Build history of the part. All positions in model axes, mm. A direction names the side the tool comes from. Round coordinates to 2 decimals unless told otherwise and drop trailing zeros. Order: outer loops, then holes, each group sorted by start corner. A loop starts at its lowest first (then second) coordinate and runs counter-clockwise, first axis right, second up. Notation, with made-up numbers: (26, 67) -> (33, 67) arc R23 cw to (33, 106) -> close; hole circle Ø11 at (14.5, 88). An arc over 180 degrees is marked (long way). Use a Markdown table: item, result. Add a question column.
Item 1: Slice it at D-D, the plane x = 31. Give the cut face in (y, z).
Item 2: Two-plate mould, pull along X, no slides. Class faces 6 (the face through (-41, 3, 23)), 7 (the face through (-32.35, 10, 37)), 8 (the face through (0, 2, 25.5)), 9 (the face through (41.99, 2.53, 51.25)): released by +X, released by -X, zero draft, split by the parting line, or undercut.
Item 3: Slice it at B-B, the plane z = 46. Give the cut face in (x, y).
Item 4: Slice it at A-A, the plane y = 13.25. Give the cut face in (x, z).
Item 5: 3-axis set-ups, long thin cutter, end or side, ignore diameter. For faces 1 (the face through (41.99, 2.53, 22.25)), 2 (the face through (32.35, 10, 37)), 3 (the face through (-34.35, 10, 37)), 4 (the face through (-42.01, 2.53, 51.25)), 5 (the face through (-25, 2, 38)): which of +Z, -Z, +X, -X, +Y, -Y reach the whole face in a straight line?
Item 6: Pin check, flat tips, straight feed: pin 1 (1.7 mm diameter, centred on x = 39, z = 32.5, fed in from +Y); pin 2 (3 mm diameter, centred on x = -13, z = 25.5, fed in from -Y); pin 3 (5 mm diameter, centred on y = 9.5, z = 35.5, fed in from +X); pin 4 (0.9 mm diameter, centred on y = 2.5, z = 52, fed in from -X). Stop position of each tip, or through.
Item 7: Slice it at C-C, the plane x = -15. Give the cut face in (y, z).
Item 8: Probe L1, parallel to X at y = 1.55, z = 38; L2, parallel to X at y = 12.75, z = 42.5; L3, parallel to Y at x = -41.55, z = 23. List the from-to ranges inside material, lowest first.
from build123d import *

# Parameters (mm, degrees)
SKETCH_1_W          = 86
SKETCH_1_H          = 174
SKETCH_1_W_2        = 50
SKETCH_1_H_2        = 25
SKETCH_1_H_3        = 55
SKETCH_1_W_3        = 76
SKETCH_1_H_4        = 43
EXTRUDE_1_DEPTH     = 5
SKETCH_4_W          = 68.7
SKETCH_4_H          = 115
SKETCH_4_W_2        = 64.7
SKETCH_4_H_2        = 37
SKETCH_4_H_3        = 70
EXTRUDE_2_DEPTH     = 10
SKETCH_5_R          = 0.75
CUT_EXTRUDE_1_DEPTH = 122.783619588
SKETCH_7_W          = 15
SKETCH_7_H          = 8
SKETCH_7_W_2        = 26
SKETCH_7_W_3        = 5
SKETCH_7_H_2        = 10
SKETCH_7_H_3        = 12.119700025
SKETCH_7_W_4        = 6
SKETCH_7_H_4        = 5
SKETCH_7_W_5        = 7
SKETCH_7_H_5        = 21
CUT_EXTRUDE_2_DEPTH = 2
SKETCH_8_R          = 0.75
CUT_EXTRUDE_3_DEPTH = 2
CUT_EXTRUDE_START   = -84
SKETCH_8_3_R        = 0.75
CUT_EXTRUDE_4_DEPTH = 2
SKETCH_9_R          = 0.75
SKETCH_9_W          = 50
SKETCH_9_H          = 55
SKETCH_9_W_2        = 86
SKETCH_9_H_2        = 56
SKETCH_9_W_3        = 76
SKETCH_9_H_3        = 43
CUT_EXTRUDE_5_DEPTH = 123.295748086


with BuildPart() as part:
    # 草图1 → 凸台-拉伸1 (new body)
    with BuildSketch(Plane(origin=(0, 0, 0), x_dir=(1, 0, 0), z_dir=(0, 1, 0))):
        with Locations((0, -26.5)):
            Rectangle(SKETCH_1_W, SKETCH_1_H)
        with Locations((0, -38)):
            Rectangle(SKETCH_1_W_2, SKETCH_1_H_2, mode=Mode.SUBTRACT)
        with Locations((0, 23)):
            Rectangle(SKETCH_1_W_2, SKETCH_1_H_3, mode=Mode.SUBTRACT)
        with Locations((0, -87)):
            Rectangle(SKETCH_1_W_3, SKETCH_1_H_4, mode=Mode.SUBTRACT)
    extrude(amount=EXTRUDE_1_DEPTH)

    # 草图4 → 凸台-拉伸2 (add)
    with BuildSketch(Plane(origin=(0, 5, 0), x_dir=(1, 0, 0), z_dir=(0, 1, 0))):
        Rectangle(SKETCH_4_W, SKETCH_4_H)
        with Locations((0, -37)):
            Rectangle(SKETCH_4_W_2, SKETCH_4_H_2, mode=Mode.SUBTRACT)
        with Locations((0, 20.5)):
            Rectangle(SKETCH_4_W_2, SKETCH_4_H_3, mode=Mode.SUBTRACT)
    extrude(amount=EXTRUDE_2_DEPTH)

    # 草图5 → 切除-拉伸1 (cut, through all)
    with BuildSketch(Plane(origin=(0, 5, 0), x_dir=(1, 0, 0), z_dir=(0, 1, 0))):
        with Locations(Location((-39, 20.5, 0), (0, 0, 270))):
            Circle(SKETCH_5_R)
        with Locations(Location((39, 20.5, 0), (0, 0, 270))):
            Circle(SKETCH_5_R)
        with Locations(Location((-39, -32.5, 0), (0, 0, 270))):
            Circle(SKETCH_5_R)
        with Locations(Location((39, -32.5, 0), (0, 0, 270))):
            Circle(SKETCH_5_R)
        with Locations(Location((-40.1427775, -60.35, 0), (0, 0, 270))):
            Circle(SKETCH_5_R)
        with Locations(Location((40.1427775, -60.35, 0), (0, 0, 270))):
            Circle(SKETCH_5_R)
        with Locations(Location((-40.1427775, -110.530299975, 0), (0, 0, 270))):
            Circle(SKETCH_5_R)
        with Locations(Location((40.1427775, -110.530299975, 0), (0, 0, 270))):
            Circle(SKETCH_5_R)
        with Locations(Location((-40.5, 57.5, 0), (0, 0, 270))):
            Circle(SKETCH_5_R)
        with Locations(Location((-40.5, -38, 0), (0, 0, 270))):
            Circle(SKETCH_5_R)
        with Locations(Location((-40.5, -85.5, 0), (0, 0, 270))):
            Circle(SKETCH_5_R)
        with Locations(Location((40.5, 57.5, 0), (0, 0, 270))):
            Circle(SKETCH_5_R)
        with Locations(Location((40.5, -38, 0), (0, 0, 270))):
            Circle(SKETCH_5_R)
        with Locations(Location((40.5, -85.5, 0), (0, 0, 270))):
            Circle(SKETCH_5_R)
        with Locations(Location((-40.5, -4.5, 0), (0, 0, 270))):
            Circle(SKETCH_5_R)
        with Locations(Location((40.5, -4.5, 0), (0, 0, 270))):
            Circle(SKETCH_5_R)
    extrude(amount=-CUT_EXTRUDE_1_DEPTH, mode=Mode.SUBTRACT)

    # 草图7 → 切除-拉伸2 (cut)
    with BuildSketch(Plane(origin=(0, 5, 0), x_dir=(1, 0, 0), z_dir=(0, 1, 0))):
        with Locations((-24.5, -61.5)):
            Rectangle(SKETCH_7_W, SKETCH_7_H)
        with Locations((0, -61.5)):
            Rectangle(SKETCH_7_W_2, SKETCH_7_H)
        with Locations((-40.5, -78.5)):
            Rectangle(SKETCH_7_W_3, SKETCH_7_H_2)
        with Locations((-40.5, -101.440149988)):
            Rectangle(SKETCH_7_W_3, SKETCH_7_H_3)
        with Locations((-32, -111)):
            Rectangle(SKETCH_7_W_4, SKETCH_7_H_4)
        with Locations((-3, -111)):
            Rectangle(SKETCH_7_W_4, SKETCH_7_H_4)
        with Locations((17.5, -111)):
            Rectangle(SKETCH_7_W_5, SKETCH_7_H_4)
        with Locations((30.5, -111)):
            Rectangle(SKETCH_7_W_5, SKETCH_7_H_4)
        with Locations((40.5, -92)):
            Rectangle(SKETCH_7_W_3, SKETCH_7_H_5)
    extrude(amount=-CUT_EXTRUDE_2_DEPTH, mode=Mode.SUBTRACT)

    # 草图8 → 切除-拉伸3 (cut)
    with BuildSketch(Plane.ZY.offset(43)):
        with Locations((8, 2.5)):
            Circle(SKETCH_8_R)
        with Locations((23, 2.5)):
            Circle(SKETCH_8_R)
        with Locations((52, 2.5)):
            Circle(SKETCH_8_R)
        with Locations((63, 2.5)):
            Circle(SKETCH_8_R)
    extrude(amount=-CUT_EXTRUDE_3_DEPTH, mode=Mode.SUBTRACT)

    # 草图8<3> → 切除-拉伸4 (cut)
    with BuildSketch(Plane.ZY.offset(43).offset(CUT_EXTRUDE_START)):
        with Locations((8, 2.5)):
            Circle(SKETCH_8_3_R)
        with Locations((23, 2.5)):
            Circle(SKETCH_8_3_R)
        with Locations((52, 2.5)):
            Circle(SKETCH_8_3_R)
        with Locations((63, 2.5)):
            Circle(SKETCH_8_3_R)
    extrude(amount=-CUT_EXTRUDE_4_DEPTH, mode=Mode.SUBTRACT)

    # 草图9 → 切除-拉伸5 (cut, through all)
    # profile 1 of 2: a face of its own
    with BuildSketch(Plane(origin=(0, 0, 0), x_dir=(1, 0, 0), z_dir=(0, 1, 0))):
        Polygon((-43, 60.5), (-43, -16.5), (0, -16.5), (43, -16.5), (43, 60.5), align=None)
        with Locations((-40.5, -4.5)):
            Circle(SKETCH_9_R, mode=Mode.SUBTRACT)
        with Locations((-39, 20.5)):
            Circle(SKETCH_9_R, mode=Mode.SUBTRACT)
        with Locations((-40.5, 57.5)):
            Circle(SKETCH_9_R, mode=Mode.SUBTRACT)
        with Locations((0, 23)):
            Rectangle(SKETCH_9_W, SKETCH_9_H, mode=Mode.SUBTRACT)
        with Locations((40.5, -4.5)):
            Circle(SKETCH_9_R, mode=Mode.SUBTRACT)
        with Locations((39, 20.5)):
            Circle(SKETCH_9_R, mode=Mode.SUBTRACT)
        with Locations((40.5, 57.5)):
            Circle(SKETCH_9_R, mode=Mode.SUBTRACT)
    # profile 2 of 2: a face of its own
    with BuildSketch(Plane(origin=(0, 0, 0), x_dir=(1, 0, 0), z_dir=(0, 1, 0))):
        with Locations((0, -85.5)):
            Rectangle(SKETCH_9_W_2, SKETCH_9_H_2)
        with Locations((-40.1427775, -110.530299975)):
            Circle(SKETCH_9_R, mode=Mode.SUBTRACT)
        with Locations((-40.5, -85.5)):
            Circle(SKETCH_9_R, mode=Mode.SUBTRACT)
        with Locations((0, -87)):
            Rectangle(SKETCH_9_W_3, SKETCH_9_H_3, mode=Mode.SUBTRACT)
        with Locations((-40.1427775, -60.35)):
            Circle(SKETCH_9_R, mode=Mode.SUBTRACT)
        with Locations((40.1427775, -110.530299975)):
            Circle(SKETCH_9_R, mode=Mode.SUBTRACT)
        with Locations((40.5, -85.5)):
            Circle(SKETCH_9_R, mode=Mode.SUBTRACT)
        with Locations((40.1427775, -60.35)):
            Circle(SKETCH_9_R, mode=Mode.SUBTRACT)
    extrude(amount=CUT_EXTRUDE_5_DEPTH, mode=Mode.SUBTRACT)


solid = part.part
Check sheet entries:
| question | item | result |
|---|---|---|
| 1 | outline | (0, 16.5) -> (15, 16.5) -> (15, 18.5) -> (5, 18.5) -> (5, 55.5) -> (15, 55.5) -> (15, 57.5) -> (0, 57.5) -> close |
| 2 | face 6 | released by -X |
| 2 | face 7 | undercut |
| 2 | face 8 | undercut |
| 2 | face 9 | zero draft |
| 3 | outline | (-43, 0) -> (-25, 0) -> (-25, 5) -> (-32.35, 5) -> (-32.35, 15) -> (-34.35, 15) -> (-34.35, 5) -> (-43, 5) -> close; (25, 0) -> (43, 0) -> (43, 5) -> (34.35, 5) -> (34.35, 15) -> (32.35, 15) -> (32.35, 5) -> (25, 5) -> close |
| 4 | outline | (-34.35, 16.5) -> (34.35, 16.5) -> (34.35, 57.5) -> (-34.35, 57.5) -> close; hole (-32.35, 18.5) -> (32.35, 18.5) -> (32.35, 55.5) -> (-32.35, 55.5) -> close |
| 5 | face 1 | +X |
| 5 | face 2 | +Y |
| 5 | face 3 | +Z, -Z, -X, +Y |
| 5 | face 4 | -X |
| 5 | face 5 | +Y, -Y |
| 6 | pin 1 | y = 5 |
| 6 | pin 2 | y = 0 |
| 6 | pin 3 | x = 34.35 |
| 6 | pin 4 | x = -41 |
| 7 | outline | (0, 16.5) -> (15, 16.5) -> (15, 18.5) -> (5, 18.5) -> (5, 25.5) -> (0, 25.5) -> close; (0, 50.5) -> (5, 50.5) -> (5, 55.5) -> (15, 55.5) -> (15, 57.5) -> (0, 57.5) -> close |
| 8 | L1 | -43 to -41.25, -39.75 to -25, 25 to 39.75, 41.25 to 43 |
| 8 | L2 | -34.35 to -32.35, 32.35 to 34.35 |
| 8 | L3 | 0 to 1.75, 3.25 to 5 |
